Part model, mm, in its own coordinate system. A direction names the side the tool comes from. Give positions to 0.01 mm unless a question says otherwise; leave off trailing zeros. Write each loop counter-clockwise with the first axis right and the second up, starting at its lowest first coordinate (ties: lowest second). Pieces come first, ordered by that corner, then holes. Notation, with made-up numbers: (45.5, -30) - (79.5, -30) arc R13 ccw to (79.5, -12) - close; hole circle Ø2 at (86.5, 39). An arc over 180 degrees is marked (long way). Answer as a JSON object with one key per item and string values. Group by question number.
```python
from build123d import *

# Parameters (mm, degrees)
BOSS_EXTRUDE1_DEPTH = 1
BOSS_EXTRUDE2_DEPTH = 1
BOSS_EXTRUDE3_DEPTH = 10
CUT_EXTRUDE1_DEPTH  = 6.35
FILLET1_R           = 1
FILLET2_R           = 0.5


with BuildPart() as part:
    # Sketch1 → Boss-Extrude1 (new body)
    with BuildSketch(Plane.XY):
        Polygon((-18.007564672, 19.736677749), (-18.007564672, -19.727423866), (-11.433074418, -31.219203109), (11.416925582, -31.219203109), (18.007564672, -19.736677749), (18.007564672, 19.727423866), (11.433074418, 31.219203109), (-11.416925582, 31.219203109), align=None)
    extrude(amount=BOSS_EXTRUDE1_DEPTH)

    # Sketch2 → Boss-Extrude2 (add)
    with BuildSketch(Plane.XY.offset(1)):
        Polygon((-10.982642952, 30.469203109), (-17.257564672, 19.536735589), (-17.257564672, -19.528046249), (-10.99808756, -30.469203109), (10.982642952, -30.469203109), (17.257564672, -19.536735589), (17.257564672, 19.528046249), (10.99808756, 30.469203109), align=None)
        Polygon((-10.114077691, 28.969203109), (-15.757564672, 19.136851269), (-15.757564672, -19.129291014), (-10.128113844, -28.969203109), (10.114077691, -28.969203109), (15.757564672, -19.136851269), (15.757564672, 19.129291014), (10.128113844, 28.969203109), align=None, mode=Mode.SUBTRACT)
    extrude(amount=BOSS_EXTRUDE2_DEPTH)

    # Sketch3 → Boss-Extrude3 (add)
    with BuildSketch(Plane.XY.offset(1)):
        Polygon((-14.2, -21.8), (-14.2, -15.3), (-12.7, -15.3), (-12.7, -20.3), (-7.7, -20.3), (-7.7, -21.8), align=None)
        Polygon((-12.7, 20.3), (-7.7, 20.3), (-7.7, 21.8), (-14.2, 21.8), (-14.2, 15.3), (-12.7, 15.3), align=None)
        Polygon((12.7, -20.3), (12.7, -15.3), (14.2, -15.3), (14.2, -21.8), (7.7, -21.8), (7.7, -20.3), align=None)
        Polygon((12.7, 15.3), (14.2, 15.3), (14.2, 21.8), (7.7, 21.8), (7.7, 20.3), (12.7, 20.3), align=None)
    extrude(amount=BOSS_EXTRUDE3_DEPTH)

    # Sketch4 → Cut-Extrude1 (cut)
    with BuildSketch(Plane.XY.offset(1)):
        Polygon((13.897999946, 35.469203109), (-13.877860488, 35.469203109), (-22.257564672, 20.869683322), (-22.257564672, -20.857230366), (-13.897999946, -35.469203109), (13.877860488, -35.469203109), (22.257564672, -20.869683322), (22.257564672, 20.857230366), align=None)
        Polygon((10.99808756, 30.469203109), (-10.982642952, 30.469203109), (-17.257564672, 19.536735589), (-17.257564672, -19.528046249), (-10.99808756, -30.469203109), (10.982642952, -30.469203109), (17.257564672, -19.536735589), (17.257564672, 19.528046249), align=None, mode=Mode.SUBTRACT)
    extrude(amount=-CUT_EXTRUDE1_DEPTH, mode=Mode.SUBTRACT)

    # Fillet1
    fillet1_edges = [part.edges().sort_by_distance(p)[0] for p in [
        (-7.7, 21.8, 6),
        (-14.2, 21.8, 6),
        (-14.2, 15.3, 6),
        (7.7, -21.8, 6),
        (14.2, -21.8, 6),
        (14.2, -15.3, 6),
        (14.2, 15.3, 6),
        (14.2, 21.8, 6),
        (7.7, 21.8, 6),
        (-14.2, -15.3, 6),
        (-14.2, -21.8, 6),
        (-7.7, -21.8, 6),
    ]]
    fillet(fillet1_edges, radius=FILLET1_R)

    # Fillet2
    fillet2_edges = [part.edges().sort_by_distance(p)[0] for p in [
        (0.007722304, 30.469203109, 2),
        (-14.120103812, 25.002969349, 2),
        (-17.257564672, 0.00434467, 2),
        (-14.127826116, -24.998624679, 2),
        (-0.007722304, -30.469203109, 2),
        (14.120103812, -25.002969349, 2),
        (17.257564672, -0.00434467, 2),
        (14.127826116, 24.998624679, 2),
    ]]
    fillet(fillet2_edges, radius=FILLET2_R)


solid = part.part
```
1) Which spindle directions (+Z, -Z, +X, -X, +Y, -Y) get a long thin tool onto all of the face, cutting with end or side? Do faces 1 (the flat face through (-14.076, 25.079, 0.76)), 2 (the flat face through (12.896, -24.122, 1.493)). Say none if no direction does.
2) Saw through at B-B (x = -6). List the corners of the cut face in (y, z).
3) Two-plate mould, pull along Y, no slides. Class faces 3 (the flat face through (-12.982, -23.98, 1.493)), 4 (the cylindrical face through (-13.95, -25, 1.86)), 5 (the cylindrical face through (13.95, 25, 1.86)), 6 (the flat face through (17.258, 0, 1)): +Y half, -Y half, draft (parallel to the pull), parting line (faces both ways), or undercut.
4) Drop flat-ended pins along their axis: P1, Ø2.5, axis at x = 9.5, z = 5.5, coming from the +Y side; P2, Ø6, axis at x = 13.5, y = -7.5, coming from the +Z side; P3, Ø5, axis at x = -2.5, y = -24, coming from the +Z side. Give the stop position or say it passes through.
5) Saw through at D-D (y = -18.5). List the corners of the cut face in (x, z).
6) Saw through at C-C (z = 6). State how many separate pieces and enclosed holes the cut face has, and give its area (3 significant figures).
7) Saw through at A-A (y = -3). List the corners of the cut face in (x, z), and give its area (3 significant figures).
8) Drill centre lines: line 1 along Y through (x, z) = (-11.5, 6.5); line 2 along Z through (x, y) = (5, 20); line 3 along X through (y, z) = (-16, 2.5). Where is each one in solid material? Low to high. Write a range as from..to.
Checks:
{
 "1": {"face 1": "+Z, -Z, -X, +Y", "face 2": "+Z"},
 "2": {"outline": "(-30.47, 0) - (30.47, 0) - (30.47, 1.5) arc R0.5 ccw to (29.97, 2) - (28.97, 2) - (28.97, 1) - (-28.97, 1) - (-28.97, 2) - (-29.97, 2) arc R0.5 ccw to (-30.47, 1.5) - close"},
 "3": {"face 3": "undercut", "face 4": "-Y half", "face 5": "+Y half", "face 6": "draft"},
 "4": {"P1": "y = 21.8", "P2": "z = 2", "P3": "z = 1"},
 "5": {"outline": "(-17.26, 0) - (17.26, 0) - (17.26, 1.5) arc R0.5 ccw to (16.76, 2) - (15.76, 2) - (15.76, 1) - (14.2, 1) - (14.2, 11) - (12.7, 11) - (12.7, 1) - (-12.7, 1) - (-12.7, 11) - (-14.2, 11) - (-14.2, 1) - (-15.76, 1) - (-15.76, 2) - (-16.76, 2) arc R0.5 ccw to (-17.26, 1.5) - close"},
 "6": {"separate pieces": "4", "enclosed holes": "0", "area": "66.4 mm2"},
 "7": {"outline": "(-17.26, 0) - (17.26, 0) - (17.26, 1.5) arc R0.5 ccw to (16.76, 2) - (15.76, 2) - (15.76, 1) - (-15.76, 1) - (-15.76, 2) - (-16.76, 2) arc R0.5 ccw to (-17.26, 1.5) - close", "area": "37.4 mm2"},
 "8": {"line 1": "-21.8..-20.3, 20.3..21.8", "line 2": "0..1", "line 3": "-14.15..-12.7, 12.7..14.15"}
}
